Geometry check sheet. Reference: the model listing, model coordinates, mm. Face numbers are marked on the shaded views. A direction names the side the tool comes from. Give positions to 0.01 mm unless a question says otherwise; leave off trailing zeros. Loops run counter-clockwise (first coordinate to the right, second up) from the corner with the lowest first, then second, coordinate; pieces in that order, holes last. Notation, with made-up numbers: (64.25, 67.25) - (84.25, 67.25) arc R14 cw to (84.25, 86.25) - close; hole circle Ø9 at (41, 51). An arc over 180 degrees is marked (long way). Use a Markdown table: item, result. Add a question column.
1. Cross-section at A-A on z = 3.75. Enter the section's corners in (x, y), and give its area (3 significant figures).
2. Depth check by flat-ended pin: P1, Ø1.5, axis at x = 92, z = 3, coming from the +Y side; P2, Ø1.5, axis at y = 77, z = 8, coming from the +X side; P3, Ø2, axis at y = 71.5, z = 14, coming from the +X side; P4, Ø16, axis at x = 84, y = 68.5, coming from the -Z side. Enter the tip coordinate at first touch or a pass-through.
3. Cross-section at C-C on y = 64.5. Enter the section's corners in (x, z), and give its area (3 significant figures).
4. Set-up check for the marked faces 1, 2 and 3: record each of +Z, -Z, +X, -X, +Y, -Y from which the full face is reachable in a straight line by a thin tool's end or side.
5. Material ranges on L1, parallel to Z at x = 83.5, y = 68; L2, parallel to Y at x = 75.75, z = 7; L3, parallel to Y at x = 92.25, z = 2, recorded low to high.
6. Cross-section at D-D on x = 86. Enter the section's corners in (y, z).
7. Cross-section at B-B on z = 14.5. Enter the section's corners in (x, y).
8. Draft check along X on the marked faces 4, 5 and 6. Enter one of: pulls with the +X half, pulls with the -X half, needs draft (parallel to the pull), parting line crosses it, or undercut.
Autodesk Inventor part; units mm, degrees
ref_plane "Work Plane1" through (72.2806, 68.9104, 57.5461) normal (0, 0, 1) x (0.7658175, 0.643058, 0)
ref_plane "Work Plane2" through (75.6298, 74.8001, 12) normal (0, 0, 1) x (0.7658175, 0.643058, 0)
ref_plane "YZ Plane" through (0, 0, 0) normal (1, 0, 0) x (0, 1, 0)
sketch "Sketch1" plane through (0, 0, 0) normal (0, 0, 1) x (1, 0, 0)
  line L0 (91.0829, 58.2221) -> (71.5983, 81.4264)
  line L1 (73.9454, 78.6312) -> (81.7568, 85.1904)
  line L2 (96.5471, 67.5766) -> (88.7358, 61.0174)
  line L3 (71.5983, 81.4264) -> (69.6691, 83.7239)
  line L4 (69.6691, 83.7239) -> (75.0298, 88.2253)
  line L5 (75.0298, 88.2253) -> (79.3061, 83.1326)
  line L6 (91.0829, 58.2221) -> (93.0121, 55.9247)
  line L7 (93.0121, 55.9247) -> (98.3728, 60.4261)
  line L8 (98.3728, 60.4261) -> (94.0965, 65.5188)
  line L9 (81.3406, 69.8243) -> (102.4069, 87.5137) construction
  line L10 (91.726, 57.4563) -> (90.0029, 56.0094)
  line L11 (95.6925, 58.1754) -> (91.4161, 63.2681) construction
  line L12 (72.3494, 85.9746) -> (76.6258, 80.8819) construction
  point P0 (0, 0)
  point P1 (93.5543, 60.7217)
  point P2 (74.4876, 83.4282)
  dimension "d0" = 2
  dimension "d1" = 7
ref_plane "Work Plane1" through (72.2806, 68.9104, 57.5461) normal (0, 0, 1) x (0.7658175, 0.643058, 0)
ref_plane "Work Plane2" through (75.6298, 74.8001, 12) normal (0, 0, 1) x (0.7658175, 0.643058, 0)
extrude "Extrusion1" add sketch "Sketch1" along normal up to surface (12 mm away)
sketch "Sketch2" plane through (98.3728, 60.4261, 12) normal (0, 0, 1) x (0.7658175, 0.643058, 0)
  line L0 (0, 0) -> (0, 6.65)
  line L1 (-7, 29.65) -> (-7, 36.3)
  line L2 (0, 0) -> (-7, 0)
  line L3 (-7, 0) -> (-7, 36.3)
  line L4 (-7, 36.3) -> (0, 36.3)
  line L5 (0, 36.3) -> (0, 0)
  point P0 (-114.1931, 16.9841)
  point P1 (0, 6.65)
  point P2 (-7, 29.65)
extrude "Extrusion2" add sketch "Sketch2" along normal blind 4
hole "Hole1" at (74.4876, 83.4282, 0) at (93.5543, 60.7217, 0) direction (0, 0, 1) diameter 3.4 end through all
fillet "Fillet1" radius 2 8 edges at (93.0121, 55.9247, 14) (93.0121, 55.9247, 6) (98.3728, 60.4261, 14) (98.3728, 60.4261, 6) (75.0298, 88.2253, 14) (75.0298, 88.2253, 6) (69.6691, 83.7239, 14) (69.6691, 83.7239, 6)
sketch "Sketch3" plane through (98.3728, 60.4261, 16) normal (0, 0, 1) x (0.7658175, 0.643058, 0)
  circle A0 centre (-3.5, 3.325) radius 1.7
  circle A1 centre (-3.5, 32.975) radius 1.7
  line L0 (-1.9123, 6.075) -> (-0.3246, 3.325)
  line L1 (-0.3246, 3.325) -> (-1.9123, 0.575)
  line L2 (-1.9123, 0.575) -> (-5.0877, 0.575)
  line L3 (-5.0877, 0.575) -> (-6.6754, 3.325)
  line L4 (-6.6754, 3.325) -> (-5.0877, 6.075)
  line L5 (-5.0877, 6.075) -> (-1.9123, 6.075)
  line L6 (-1.9123, 30.225) -> (-5.0877, 30.225)
  line L7 (-5.0877, 30.225) -> (-6.6754, 32.975)
  line L8 (-6.6754, 32.975) -> (-5.0877, 35.725)
  line L9 (-5.0877, 35.725) -> (-1.9123, 35.725)
  line L10 (-1.9123, 35.725) -> (-0.3246, 32.975)
  line L11 (-0.3246, 32.975) -> (-1.9123, 30.225)
  line L12 (-5, 0) -> (-2, 0)
  point P0 (-114.1931, 16.9841)
  point P1 (-3.5, 3.325)
  point P2 (-3.5, 32.975)
  dimension "d14" = 5.5
  dimension "d15" = 5.5
extrude "Extrusion3" cut sketch "Sketch3" against normal blind 2
properties part number "servo_holder"
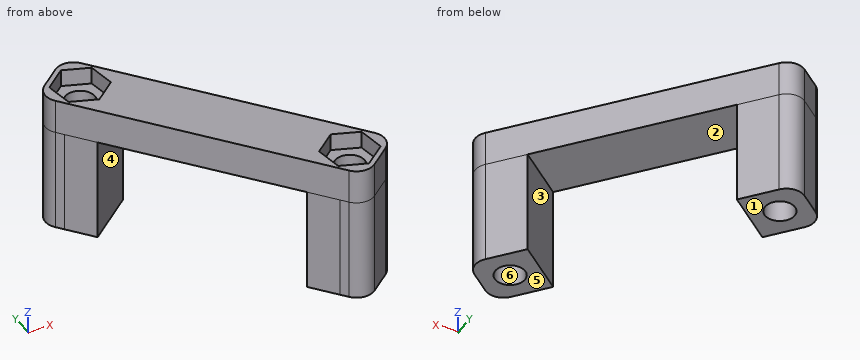
Values found:
| question | item | result |
|---|---|---|
| 1 | outline | (70.96, 82.19) - (71.6, 81.43) - (73.95, 78.63) - (79.31, 83.13) - (76.32, 86.69) arc R2 ccw to (73.5, 86.94) - (71.2, 85.01) arc R2 ccw to start; (88.74, 61.02) - (91.08, 58.22) - (91.73, 57.46) arc R2 ccw to (94.54, 57.21) - (96.84, 59.14) arc R2 ccw to (97.09, 61.96) - (94.1, 65.52) - close; hole circle Ø3.4 at (74.49, 83.43); hole circle Ø3.4 at (93.55, 60.72) |
| 1 | area | 71.5 mm2 |
| 2 | P1 | stops at y = 64.39 |
| 2 | P2 | passes through |
| 2 | P3 | stops at x = 89.91 |
| 2 | P4 | stops at z = 12 |
| 3 | outline | (85.81, 12) - (92.88, 12) - (92.88, 0) - (94.95, 0) - (94.95, 16) - (85.81, 16) - close |
| 3 | area | 61.4 mm2 |
| 4 | face 1 | -Z, +X, -X, +Y, -Y |
| 4 | face 2 | -Z |
| 4 | face 3 | -Z, -X, +Y |
| 5 | L1 | z = 12 to 16 |
| 5 | L2 | y = 80.15 to 82.29, 84.57 to 87.16 |
| 5 | L3 | y = 57.01 to 59.63, 61.81 to 63.97 |
| 6 | outline | (64.28, 12) - (75.16, 12) - (75.16, 16) - (64.28, 16) - close |
| 7 | outline | (70.96, 82.19) - (91.73, 57.46) arc R2 ccw to (94.54, 57.21) - (96.84, 59.14) arc R2 ccw to (97.09, 61.96) - (76.32, 86.69) arc R2 ccw to (73.5, 86.94) - (71.2, 85.01) arc R2 ccw to start; hole (71.5, 84.51) - (72.06, 81.39) - (75.04, 80.3) - (77.47, 82.34) - (76.92, 85.47) - (73.94, 86.56) - close; hole (90.57, 61.81) - (91.12, 58.68) - (94.11, 57.59) - (96.54, 59.64) - (95.99, 62.76) - (93, 63.85) - close |
| 8 | face 4 | pulls with the +X half |
| 8 | face 5 | needs draft |
| 8 | face 6 | undercut |
